Build history of the part. All positions in model axes, mm. A direction names the side the tool comes from. Coordinates: 2 decimals unless noted, no trailing zeros. Order: outer loops, then holes, each group sorted by start corner. A loop starts at its lowest first (then second) coordinate and runs counter-clockwise, first axis right, second up. Notation, with made-up numbers: M 88,38.5 L 130,38.5 A28 cw 130,63.5 Z; hole C -39.5,21.5 d4. An arc over 180 degrees is marked long. Write item = value, one per line. Start each with the question number.
Q1. Pull direction X, two halves, no side cores. Call faces 1 (the face through (25.4, 16, 23)), 2 (the face through (13, 50.8, 24)), 3 (the face through (10.18, 36.17, 23.83)): released by +X, released by -X, zero draft, split by the parting line, or undercut.
Q2. Pin check, flat tips, straight feed: P1, Ø10, axis at x = 10, z = 5, coming from the +Y side (3 decimals); P2, Ø7.5, axis at x = 13.5, y = 30.5, coming from the -Z side (3 decimals). Stop position of each tip, or through.
Q3. Band-saw the part on D-D on z = 5. Write the cut outline in (x, y) (3 decimals).
Q4. 3-axis set-ups, long thin cutter, end or side, ignore diameter. For faces 4 (the face through (0, 16, 23)), 5 (the face through (15, 3.175, 12)): which of +Z, -Z, +X, -X, +Y, -Y reach the whole face in a straight line?
Q5. Drill centre lines: probe 1 along Y at (x, z) = (12.7, 24.15) (3 decimals); probe 2 along Z at (x, y) = (6.25, 28.5) (3 decimals); probe 3 along Y at (x, z) = (12.7, 23) (3 decimals). Where is each one in solid material? Low to high.
Q6. Band-saw the part on B-B on y = 19.05. Write the cut outline in (x, z) (3 decimals), plus the area to 3 significant figures.
Q7. Band-saw the part on C-C on x = 22.25. Write the cut outline in (y, z) (3 decimals).
Q8. Band-saw the part on A-A on x = 12.7. Write the cut outline in (y, z) (3 decimals).
```python
from build123d import *

# Parameters (mm, degrees)
BASE_FLANGE1_DEPTH              = 25.4
F_1_4_0_25_DIAMETER_HOLE1_D     = 6.35
F_1_4_0_25_DIAMETER_HOLE1_DEPTH = 10.7188
F_1_4_0_25_DIAMETER_HOLE1_TIP   = 1.907732465
F_1_4_0_25_DIAMETER_HOLE2_D     = 6.35
F_1_4_0_25_DIAMETER_HOLE2_DEPTH = 10.7188
F_1_4_0_25_DIAMETER_HOLE2_TIP   = 1.907732465


# Sheet-metal steps are written as plain solids
with BuildPart() as part:
    # Sketch1 → Base-Flange1 (new body)
    with BuildSketch(Plane(origin=(0, 0, 0), x_dir=(0, 0, -1), z_dir=(1, 0, 0))):
        with BuildLine():
            Line((0, 0), (-19.05, 0))
            ThreePointArc((-19.05, 0), (-23.540128061, 1.859871939), (-25.4, 6.35))
            Line((-25.4, 6.35), (-25.4, 50.8))
            Line((-25.4, 50.8), (-22.225, 50.8))
            Line((-22.225, 50.8), (-22.225, 6.35))
            ThreePointArc((-22.225, 6.35), (-21.29506403, 4.10493597), (-19.05, 3.175))
            Line((-19.05, 3.175), (0, 3.175))
            Line((0, 3.175), (0, 0))
        make_face()
    extrude(amount=BASE_FLANGE1_DEPTH)

    # 1/4 (0.25) Diameter Hole1
    with Locations(Plane(origin=(0, 0, 22.225), x_dir=(-1, 0, 0), z_dir=(0, 0, -1))):
        with Locations((-12.7, 38.1), (-12.7, 19.05)):
            Hole(F_1_4_0_25_DIAMETER_HOLE1_D / 2, depth=F_1_4_0_25_DIAMETER_HOLE1_DEPTH)
            with Locations((0, 0, -(F_1_4_0_25_DIAMETER_HOLE1_DEPTH + F_1_4_0_25_DIAMETER_HOLE1_TIP / 2))):  # 118° drill point
                Cone(0, F_1_4_0_25_DIAMETER_HOLE1_D / 2, F_1_4_0_25_DIAMETER_HOLE1_TIP, mode=Mode.SUBTRACT)

    # 1/4 (0.25) Diameter Hole2
    with Locations(Plane(origin=(0, 3.175, 0), x_dir=(1, 0, 0), z_dir=(0, 1, 0))):
        with Locations((12.7, -9.525)):
            Hole(F_1_4_0_25_DIAMETER_HOLE2_D / 2, depth=F_1_4_0_25_DIAMETER_HOLE2_DEPTH)
            with Locations((0, 0, -(F_1_4_0_25_DIAMETER_HOLE2_DEPTH + F_1_4_0_25_DIAMETER_HOLE2_TIP / 2))):  # 118° drill point
                Cone(0, F_1_4_0_25_DIAMETER_HOLE2_D / 2, F_1_4_0_25_DIAMETER_HOLE2_TIP, mode=Mode.SUBTRACT)


solid = part.part
```
Recorded:
q1.face_1 = released by +X
q1.face_2 = zero draft
q1.face_3 = undercut
q2.P1 = 3.175
q2.P2 = 22.225
q3.outline = M 0,0 L 25.4,0 L 25.4,3.175 L 0,3.175 Z
q4.face_4 = +Z, -Z, -X, +Y, -Y
q4.face_5 = -Z, +X, -X, +Y
q5.probe_1 = 2.567 to 15.875, 22.225 to 34.925, 41.275 to 50.8
q5.probe_2 = 22.225 to 25.4
q5.probe_3 = 1.378 to 15.875, 22.225 to 34.925, 41.275 to 50.8
q6.outline = M 0,22.225 L 9.525,22.225 L 9.525,25.4 L 0,25.4 Z; M 15.875,22.225 L 25.4,22.225 L 25.4,25.4 L 15.875,25.4 Z
q6.area = 60.5 mm2
q7.outline = M 0,0 L 3.175,0 L 3.175,19.05 A3.175 cw 6.35,22.225 L 50.8,22.225 L 50.8,25.4 L 6.35,25.4 A6.35 ccw 0,19.05 Z
q8.outline = M 0,0 L 3.175,0 L 3.175,6.35 L 0,6.35 Z; M 0,12.7 L 3.175,12.7 L 3.175,19.05 A3.175 cw 6.35,22.225 L 15.875,22.225 L 15.875,25.4 L 6.35,25.4 A6.35 ccw 0,19.05 Z; M 22.225,22.225 L 34.925,22.225 L 34.925,25.4 L 22.225,25.4 Z; M 41.275,22.225 L 50.8,22.225 L 50.8,25.4 L 41.275,25.4 Z
